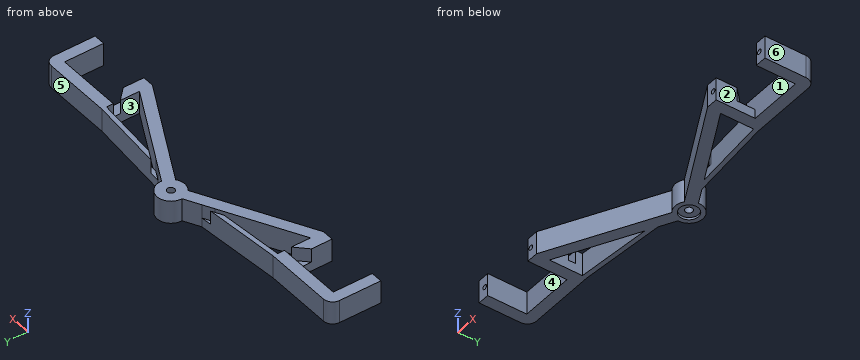
from build123d import *

# Parameters (mm, degrees)
SKETCH1_R           = 8
BOSS_EXTRUDE1_DEPTH = 25
CUT_EXTRUDE1_START  = 85
SKETCH2_R           = 5.25
CUT_EXTRUDE1_DEPTH  = 30
FILLET1_R           = 20
BOSS_EXTRUDE2_DEPTH = 50
CUT_EXTRUDE2_DEPTH  = 30
SKETCH5_R           = 20.5
CUT_EXTRUDE3_DEPTH  = 5


with BuildPart() as part:
    # Sketch1 → Boss-Extrude1 (new, symmetric)
    with BuildSketch(Plane.XY):
        with BuildLine():
            Line((25, 85), (25, 0))
            Line((25, 0), (0, 0))
            Line((0, 0), (0, 110))
            Line((0, 110), (167.5, 110))
            Line((167.5, 110), (167.5, 28.258760447))
            Line((167.5, 28.258760447), (387.545711729, 144.215139733))
            ThreePointArc((387.545711729, 144.215139733), (417.5, 175.870619777), (447.454288271, 144.215139733))
            Line((447.454288271, 144.215139733), (667.5, 28.258760447))
            Line((667.5, 28.258760447), (667.5, 110))
            Line((667.5, 110), (835, 110))
            Line((835, 110), (835, 0))
            Line((835, 0), (810, 0))
            Line((810, 0), (810, 85))
            Line((810, 85), (692.5, 85))
            Line((692.5, 85), (692.5, 0))
            Line((692.5, 0), (667.5, 0))
            Line((667.5, 0), (435.799385732, 122.098104516))
            ThreePointArc((435.799385732, 122.098104516), (417.5, 115.870619777), (399.200614268, 122.098104516))
            Line((399.200614268, 122.098104516), (167.5, 0))
            Line((167.5, 0), (142.5, 0))
            Line((142.5, 0), (142.5, 85))
            Line((142.5, 85), (25, 85))
        make_face()
        with Locations((417.5, 145.870619777)):
            Circle(SKETCH1_R, mode=Mode.SUBTRACT)
    extrude(amount=BOSS_EXTRUDE1_DEPTH, both=True)

    # Sketch2 → Cut-Extrude1 (cut)
    with BuildSketch(Plane.XZ.offset(-85).offset(CUT_EXTRUDE1_START)):
        with Locations(Location((16.275, 0, 0), (0, 0, 90))):
            Circle(SKETCH2_R)
        with Locations(Location((151.225, 0, 0), (0, 0, 90))):
            Circle(SKETCH2_R)
        with Locations(Location((683.775, 0, 0), (0, 0, 90))):
            Circle(SKETCH2_R)
        with Locations(Location((818.725, 0, 0), (0, 0, 90))):
            Circle(SKETCH2_R)
    extrude(amount=-CUT_EXTRUDE1_DEPTH, mode=Mode.SUBTRACT)

    # Fillet1
    fillet1_edges = [part.edges().sort_by_distance(p)[0] for p in [
        (0, 110, 0),
        (835, 110, 0),
    ]]
    fillet(fillet1_edges, radius=FILLET1_R)

    # Sketch3 → Boss-Extrude2 (add)
    with BuildSketch(Plane.XY.offset(25)):
        Polygon((353.496925298, 126.272622414), (167.5, 110), (167.5, 99.961801625), (330.655651498, 114.236071521), align=None)
        Polygon((667.5, 110), (481.503074702, 126.272622414), (504.344348502, 114.236071521), (667.5, 99.961801625), align=None)
    extrude(amount=-BOSS_EXTRUDE2_DEPTH)

    # Sketch4 → Cut-Extrude2 (cut)
    with BuildSketch(Plane.XY.offset(25)):
        Polygon((142.5, 85), (167.5, 85), (167.5, 70), (142.5, 45), align=None)
        Polygon((330.655651498, 114.236071521), (353.496925298, 126.272622414), (330.348569212, 124.247403677), (307.507295412, 112.210852784), align=None)
        Polygon((527.492704588, 112.210852784), (504.344348502, 114.236071521), (481.503074702, 126.272622414), (504.651430788, 124.247403677), align=None)
        Polygon((692.5, 45), (692.5, 85), (667.5, 85), (667.5, 70), align=None)
    extrude(amount=-CUT_EXTRUDE2_DEPTH, mode=Mode.SUBTRACT)

    # Sketch5 → Cut-Extrude3 (cut)
    with BuildSketch(Plane(origin=(0, 0, -25), x_dir=(-1, 0, 0), z_dir=(0, 0, -1))):
        with Locations((-417.5, 145.870619777)):
            Circle(SKETCH5_R)
    extrude(amount=-CUT_EXTRUDE3_DEPTH, mode=Mode.SUBTRACT)


solid = part.part
Input: part model. Units: mm. Frame: model coordinates. Face numbers are marked on the shaded views. A direction names the side the tool comes from. Coordinates: 2 decimals unless noted, no trailing zeros. Loops run counter-clockwise (first coordinate to the right, second up) from the corner with the lowest first, then second, coordinate; pieces in that order, holes last. Notation, with made-up numbers: (15, 55) -> (67, 55) arc R16 ccw to (67, 71) -> close; hole circle Ø2 at (12.25, 68). An arc over 180 degrees is marked (long way). One line per item, written item: value.
(1) Cut plane D-D (x = 612.5). Output: boundary loops of the cut face in (y, z).
Answer below:
outline: (28.98, -25) -> (57.24, -25) -> (57.24, 25) -> (28.98, 25) -> close; (104.77, -25) -> (114.81, -25) -> (114.81, 25) -> (104.77, 25) -> close
(2) Ray query, line 1 along Y through (x, z) = (417, -22); line 2 along X through (y, z) = (44, 14.5); line 3 along X through (y, z) = (83.5, -1.5). Return the intervals inside material, ascending.
Answer below:
line 1: y = 115.87 to 125.38, 166.36 to 175.87
line 2: x = 0 to 25, 142.5 to 167.5, 197.37 to 251, 584 to 637.63, 667.5 to 692.5, 810 to 835
line 3: x = 0 to 25, 272.33 to 325.95, 509.05 to 562.67, 810 to 835
(3) Cut plane A-A (x = 417.5). Output: boundary loops of the cut face in (y, z).
Answer below:
outline: (115.87, -25) -> (125.37, -25) -> (125.37, -20) -> (137.87, -20) -> (137.87, 25) -> (115.87, 25) -> close; (153.87, -20) -> (166.37, -20) -> (166.37, -25) -> (175.87, -25) -> (175.87, 25) -> (153.87, 25) -> close
(4) Pin query (flat end, axial travel): pin 1 Ø3 at (x, z) = (821, -2.5) entering from -Y; pin 2 Ø10 at (x, z) = (436, -16.5) entering from +Y; pin 3 Ø9.5 at (x, y) = (417.5, 145.87) entering from -Z; pin 4 Ø25 at (x, z) = (79, 10.5) entering from -Y. Return the tip coordinate at first contact, or that it passes through.
Answer below:
pin 1: stops at y = 30
pin 2: stops at y = 172.66
pin 3: passes through
pin 4: stops at y = 85
(5) Draft query along X for the marked faces 4, 5 and 6. Return one class per face: pulls with the +X half, pulls with the -X half, needs draft (parallel to the pull), parting line crosses it, or undercut.
Answer below:
face 4: undercut
face 5: needs draft
face 6: pulls with the +X half
(6) Cut plane B-B (y = 63). Output: boundary loops of the cut face in (x, z), then the cut area to 3 significant figures.
Answer below:
outline: (0, -25) -> (25, -25) -> (25, 25) -> (0, 25) -> close; (142.5, -25) -> (167.5, -25) -> (167.5, 25) -> (160.5, 25) -> (160.5, -5) -> (142.5, -5) -> close; (233.43, -25) -> (287.05, -25) -> (287.05, 25) -> (233.43, 25) -> close; (547.95, -25) -> (601.57, -25) -> (601.57, 25) -> (547.95, 25) -> close; (667.5, -25) -> (692.5, -25) -> (692.5, -5) -> (674.5, -5) -> (674.5, 25) -> (667.5, 25) -> close; (810, -25) -> (835, -25) -> (835, 25) -> (810, 25) -> close
area: 9,280 mm2
(7) Cut plane C-C (x = 718.5). Output: boundary loops of the cut face in (y, z).
Answer below:
outline: (85, -25) -> (110, -25) -> (110, 25) -> (85, 25) -> close
(8) Set-up query: the marked faces 1, 2 and 3. Return all of +Z, -Z, +X, -X, +Y, -Y with unobstructed straight access to the full face (end or side cutting, diameter ignored); none if empty.
Answer below:
face 1: +Z
face 2: +Z, -Z, -Y
face 3: +Z, -Z
